```python
from build123d import *

# Parameters (mm, degrees)
BOSS_EXTRUDE1_DEPTH      = 350
BOSS_EXTRUDE1_DEPTH_BACK = 350


with BuildPart() as part:
    # Sketch1 → Boss-Extrude1 (new, two sides: drawn at the far end of the back side and taken through both)
    with BuildSketch(Plane.XY.offset(-BOSS_EXTRUDE1_DEPTH_BACK)):
        Polygon((61, 0), (-61, 0), (-60.092059993, 26), (-58.092059993, 26), (-57.393644603, 6), (-50.790475383, 6), (-50.092059993, 26), (-48.092059993, 26), (-47.393644603, 6), (-40.790475383, 6), (-40.092059993, 26), (-38.092059993, 26), (-37.393644603, 6), (-30.790475383, 6), (-30.092059993, 26), (-28.092059993, 26), (-27.393644603, 6), (-20.790475383, 6), (-20.092059993, 26), (-18.092059993, 26), (-17.393644603, 6), (-10.790475383, 6), (-10.092059993, 26), (-8.092059993, 26), (-7.393644603, 6), (7.393644603, 6), (8.092059993, 26), (10.092059993, 26), (10.790475383, 6), (17.393644603, 6), (18.092059993, 26), (20.092059993, 26), (20.790475383, 6), (27.393644603, 6), (28.092059993, 26), (30.092059993, 26), (30.790475383, 6), (37.393644603, 6), (38.092059993, 26), (40.092059993, 26), (40.790475383, 6), (47.393644603, 6), (48.092059993, 26), (50.092059993, 26), (50.790475383, 6), (57.393644603, 6), (58.092059993, 26), (60.092059993, 26), align=None)
    extrude(amount=BOSS_EXTRUDE1_DEPTH + BOSS_EXTRUDE1_DEPTH_BACK)


solid = part.part
```
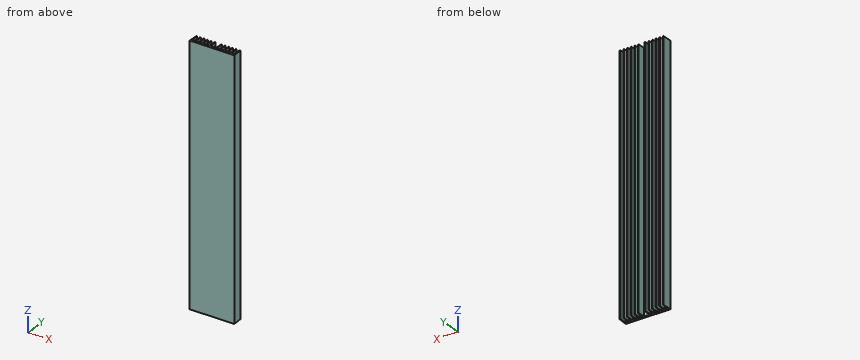
The listing builds one solid part. Answer for the finished solid, in the listing's coordinates (mm). Give positions to 0.01 mm unless a question says otherwise; leave off trailing zeros. Use one line per item in the form item = value. Start each with the question number.
1) Consider line 1 along X through (y, z) = (1.5, -299); line 2 along Y through (x, z) = (45.5, 37.5). Determine where each line is inside the solid, lowest interval first. Write a range as from..to.
2) Find section A-A on y = 14.5. Count the separate pieces of the cut face and the enclosed holes in it, plus the area to 3 significant figures.
3) Flat-ended cylindrical pins translate along their axes: pin 1 Ø2 at (y, z) = (10.5, 7.5) entering from -X; pin 2 Ø6 at (y, z) = (8.5, -226) entering from +X; pin 3 Ø2 at (x, z) = (44.5, 41) entering from +Y. Find the tip coordinate at first contact, or state that the pin passes through.
Geometry results:
q1.line_1 = -60.95..60.95
q1.line_2 = 0..6
q2.separate_pieces = 12
q2.enclosed_holes = 0
q2.area = 23,500 mm2
q3.pin_1 = -60.67
q3.pin_2 = 60.81
q3.pin_3 = 6
